Autodesk Fusion 360 part; units mm, degrees
sketch "Sketch1" plane through (0, 0, 0) normal (0, 0, 1) x (1, 0, 0)
  line L0 (39.5, 28) -> (-39.5, 28)
  line L1 (-39.5, 28) -> (-39.5, -28)
  line L2 (-39.5, -28) -> (39.5, -28)
  line L3 (39.5, -28) -> (39.5, 28)
  line L4 (39.5, 28) -> (-39.5, -28) construction
  line L5 (-39.5, 28) -> (39.5, -28) construction
  dimension "d1" = 79
  dimension "d2" = 56
extrude "Extrude1" add sketch "Sketch1" along normal blind 7
sketch "Sketch2" plane through (0, 0, 7) normal (0, 0, 1) x (-1, 0, 0)
  line L0 (-39.5, 28) -> (-39.5, -28)
  line L1 (-39.5, -28) -> (39.5, -28)
  line L2 (39.5, -28) -> (39.5, 28)
  line L3 (39.5, 28) -> (-39.5, 28)
  line L4 (-35.25, -23.75) -> (35.25, -23.75)
  line L5 (35.25, -23.75) -> (35.25, 23.75)
  line L6 (35.25, 23.75) -> (-35.25, 23.75)
  line L7 (-35.25, 23.75) -> (-35.25, -23.75)
  line L8 (-35.25, -23.75) -> (35.25, 23.75) construction
  line L9 (35.25, -23.75) -> (-35.25, 23.75) construction
  dimension "d5" = 70.5
  dimension "d6" = 47.5
extrude "Extrude2" cut sketch "Sketch2" against normal blind 3.75 contours L4 L5 L6 L7
sketch "Sketch3" plane through (0, 0, 3.25) normal (0, 0, 1) x (-1, 0, 0)
  line L0 (-35.25, 23.75) -> (-35.25, -23.75)
  line L1 (-35.25, -23.75) -> (35.25, -23.75)
  line L2 (35.25, -23.75) -> (35.25, 23.75)
  line L3 (35.25, 23.75) -> (-35.25, 23.75)
  line L4 (33.25, 21.75) -> (-33.25, 21.75)
  line L5 (-33.25, 21.75) -> (-33.25, -21.75)
  line L6 (-33.25, -21.75) -> (33.25, -21.75)
  line L7 (33.25, -21.75) -> (33.25, 21.75)
  line L8 (33.25, 21.75) -> (-33.25, -21.75) construction
  line L9 (-33.25, 21.75) -> (33.25, -21.75) construction
  dimension "d9" = 66.5
  dimension "d10" = 43.5
extrude "Extrude3" cut sketch "Sketch3" against normal blind 3.25 contours L4 L5 L6 L7
sketch "Sketch4" plane through (0, 0, 7) normal (0, 0, 1) x (-1, 0, 0)
  line L0 (35.25, -23.75) -> (-35.25, -23.75)
  line L1 (-35.25, -23.75) -> (-35.25, 23.75)
  line L2 (-35.25, 23.75) -> (35.25, 23.75)
  line L3 (35.25, 23.75) -> (35.25, -23.75)
  line L4 (-39.5, 28) -> (-39.5, -28)
  line L5 (-39.5, -28) -> (39.5, -28)
  line L6 (39.5, -28) -> (39.5, 28)
  line L7 (39.5, 28) -> (-39.5, 28)
  circle A0 centre (37.375, -25.875) radius 2
  dimension "d13" = 4
  dimension "d14" = 2.125
  dimension "d15" = 2.125
sketch "Sketch5" plane through (0, 0, 7) normal (0, 0, 1) x (-1, 0, 0)
  line L0 (35.25, -23.75) -> (-35.25, -23.75)
  line L1 (-35.25, -23.75) -> (-35.25, 23.75)
  line L2 (-35.25, 23.75) -> (35.25, 23.75)
  line L3 (35.25, 23.75) -> (35.25, -23.75)
  line L4 (-39.5, 28) -> (-39.5, -28)
  line L5 (-39.5, -28) -> (39.5, -28)
  line L6 (39.5, -28) -> (39.5, 28)
  line L7 (39.5, 28) -> (-39.5, 28)
  circle A0 centre (-37.375, -25.875) radius 2
  circle A1 centre (-37.375, 25.875) radius 2
  circle A2 centre (37.375, 25.875) radius 2
  dimension "d23" = 4
  dimension "d24" = 2.125
  dimension "d25" = 2.125
  dimension "d26" = 4
  dimension "d27" = 2.125
  dimension "d28" = 2.125
  dimension "d29" = 4
  dimension "d30" = 2.125
  dimension "d31" = 2.125
hole "Hole2" at (37.375, 25.875, 7) at (37.375, -25.875, 7) at (-37.375, -25.875, 7) direction (0, 0, -1) diameter 1.6256 depth 7.0104 tip angle 180 countersink diameter 3.9878 countersink angle 90
sketch "Sketch6" plane through (0, 0, 7) normal (0, 0, 1) x (-1, 0, 0)
  circle A0 centre (-37.375, 25.875) radius 1.9939
  circle A1 centre (-37.375, -25.875) radius 1.9939
  circle A2 centre (37.375, 25.875) radius 1.9939
  line L0 (35.25, -23.75) -> (-35.25, -23.75)
  line L1 (-35.25, -23.75) -> (-35.25, 23.75)
  line L2 (-35.25, 23.75) -> (35.25, 23.75)
  line L3 (35.25, 23.75) -> (35.25, -23.75)
  line L4 (-39.5, 28) -> (-39.5, -28)
  line L5 (-39.5, -28) -> (39.5, -28)
  line L6 (39.5, -28) -> (39.5, 28)
  line L7 (39.5, 28) -> (-39.5, 28)
  circle A3 centre (37.375, -25.875) radius 2
  dimension "d39" = 4
  dimension "d40" = 2.125
  dimension "d41" = 2.125
hole "Hole3" at (-37.375, 25.875, 7) direction (0, 0, -1) diameter 1.6256 depth 7.0104 tip angle 180 countersink diameter 3.9878 countersink angle 90
sketch "Sketch7" plane through (0, 0, 3.25) normal (0, 0, 1) x (-1, 0, 0)
  line L0 (-33.25, 21.75) -> (33.25, 21.75)
  line L1 (33.25, 21.75) -> (33.25, -21.75)
  line L2 (33.25, -21.75) -> (-33.25, -21.75)
  line L3 (-33.25, -21.75) -> (-33.25, 21.75)
  line L4 (-35.25, 23.75) -> (-35.25, -23.75)
  line L5 (-35.25, -23.75) -> (35.25, -23.75)
  line L6 (35.25, -23.75) -> (35.25, 23.75)
  line L7 (35.25, 23.75) -> (-35.25, 23.75)
sketch "Sketch8" plane through (35.25, 0, 0) normal (-1, 0, 0) x (0, -1, 0)
  line L0 (23.75, 7) -> (-23.75, 7)
  line L1 (-23.75, 7) -> (-23.75, 3.25)
  line L2 (-23.75, 3.25) -> (23.75, 3.25)
  line L3 (23.75, 3.25) -> (23.75, 7)
The model under review builds one solid part; all positions refer to its coordinate system, in mm. A direction names the side the tool comes from. Give positions to 0.01 mm unless a question says otherwise; leave off trailing zeros. Loops run counter-clockwise (first coordinate to the right, second up) from the corner with the lowest first, then second, coordinate; pieces in that order, holes last. Notation, with made-up numbers: (4, 5) -> (51, 5) arc R33 cw to (51, 43) -> close; hole circle Ø6 at (15.25, 29.25). An arc over 180 degrees is marked (long way). Put each result on its own line as item: value. Start each with the question number.
1. We need section A-A on x = -23. State the section outline as (y, z) points.
2. For faces 1 (the face through (33.25, 0, 2)), 2 (the face through (0, -23.75, 5)), 3 (the face through (-39.5, 0, 3)), list the 3-axis set-ups (+Z, -Z, +X, -X, +Y, -Y) from which the entire face can be reached by the end or side of a thin tool; tool diameter is ignored.
3. Wall thickness on probe 1 along Y at (x, z) = (-17, 2.25); probe 2 along X at (y, z) = (0, 6.5); probe 3 along X at (y, z) = (-25.5, 3): over which ranges is each line inside the solid? List them lowest first.
4. Mouldability with a two-part tool opening along Y and no side actions: class faces 4 (the face through (39.5, 0, 3)), 5 (the face through (-1, -28, 3)), 6 (the face through (0, 21.75, 2)) as released by +Y, released by -Y, zero draft, split by the parting line, or undercut.
5. We need section C-C on z = 2. State the section outline as (x, y) points (3 decimals), then the cut area to 3 significant figures.
6. We need section B-B on y = -7.5. State the section outline as (x, z) points.
7. Clearance check with flat-ended pins moving along their axes: P1, Ø1.3, axis at x = 37.375, y = -25.875, coming from the +Z side; P2, Ø1.9, axis at x = 37.375, y = 25.875, coming from the +Z side. State where each tip first meets the part, or that it passes through.
Determined:
1. outline: (-28, 0) -> (-21.75, 0) -> (-21.75, 3.25) -> (-23.75, 3.25) -> (-23.75, 7) -> (-28, 7) -> close; (21.75, 0) -> (28, 0) -> (28, 7) -> (23.75, 7) -> (23.75, 3.25) -> (21.75, 3.25) -> close
2. face 1: +Z, -Z
2. face 2: +Z
2. face 3: +Z, -Z, -X, +Y, -Y
3. probe 1: -28 to -21.75, 21.75 to 28
3. probe 2: -39.5 to -35.25, 35.25 to 39.5
3. probe 3: -39.5 to -38.1, -36.65 to 36.65, 38.1 to 39.5
4. face 4: zero draft
4. face 5: released by -Y
4. face 6: undercut
5. outline: (-39.5, -28) -> (39.5, -28) -> (39.5, 28) -> (-39.5, 28) -> close; hole circle Ø1.626 at (-37.375, -25.875); hole circle Ø1.626 at (-37.375, 25.875); hole (-33.25, -21.75) -> (33.25, -21.75) -> (33.25, 21.75) -> (-33.25, 21.75) -> close; hole circle Ø1.626 at (37.375, -25.875); hole circle Ø1.626 at (37.375, 25.875)
5. area: 1,520 mm^2
6. outline: (-39.5, 0) -> (-33.25, 0) -> (-33.25, 3.25) -> (-35.25, 3.25) -> (-35.25, 7) -> (-39.5, 7) -> close; (33.25, 0) -> (39.5, 0) -> (39.5, 7) -> (35.25, 7) -> (35.25, 3.25) -> (33.25, 3.25) -> close
7. P1: through
7. P2: z = 5.96
